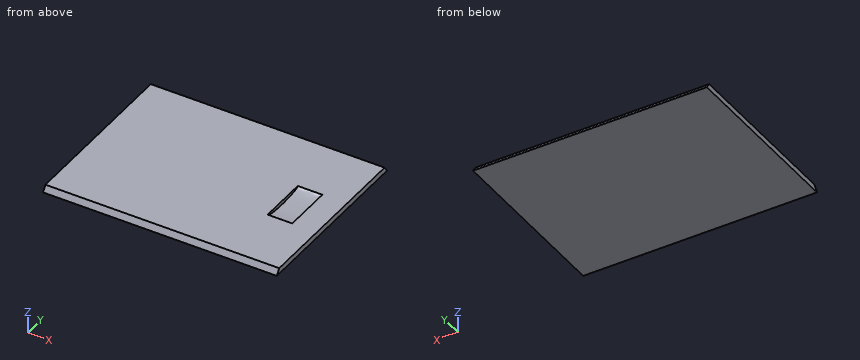
from build123d import *

# Parameters (mm, degrees)
ESBO_O1_W                = 4.6
ESBO_O1_H                = 140
RESSALTO_EXTRUS_O1_DEPTH = 190
CORTE_EXTRUS_O1_START    = -20
ESBO_O2_RX               = 20.00007904
ESBO_O2_RY               = 3.000011856
CORTE_EXTRUS_O1_DEPTH    = 20


with BuildPart() as part:
    # Esboço1 → Ressalto-extrusão1 (new body)
    with BuildSketch(Plane(origin=(0, 0, 0), x_dir=(0, 0, -1), z_dir=(1, 0, 0))):
        Rectangle(ESBO_O1_W, ESBO_O1_H)
        Polygon((2.3, 70), (-2.3, 70), (2.3, 73.220954676), align=None)
        Polygon((2.3, -70), (-2.3, -70), (2.3, -73.220954676), align=None)
    extrude(amount=RESSALTO_EXTRUS_O1_DEPTH)

    # Esboço2 → Corte-extrusão1 (cut)
    with BuildSketch(Plane(origin=(190, 0, 0), x_dir=(0, 0, -1), z_dir=(1, 0, 0)).offset(CORTE_EXTRUS_O1_START)):
        with Locations(Location((-2.3, 0), (0, 0, -89.838918547))):
            Ellipse(ESBO_O2_RX, ESBO_O2_RY)
    extrude(amount=-CORTE_EXTRUS_O1_DEPTH, mode=Mode.SUBTRACT)


solid = part.part
CAD build for the part. Positions are in the model's coordinates, mm. Round coordinates to 2 decimals unless told otherwise and drop trailing zeros. Write each loop counter-clockwise with the first axis right and the second up, starting at its lowest first coordinate (ties: lowest second). Pieces come first, ordered by that corner, then holes. Notation, with made-up numbers: M 74,28.25 L 108,28.25 A14 cw 108,48.25 Z; hole C 40.25,24 d10. An arc over 180 degrees is marked long. Use a Markdown table: item, result. Add a question column.
1. Drill centre lines: probe 1 along Y at (x, z) = (26, 1.55); probe 2 along Y at (x, z) = (123.5, 1.05); probe 3 along Z at (x, y) = (164.5, 10.5). Where is each one in solid material? Low to high.
2. Flat gauge pin, fed straight in: P1, Ø2, axis at x = 67.5, z = 0, coming from the +Y side. Where does the tip first touch, or does it go through?
3. Slice it at A-A on x = 127. Give the cut face in (y, z), then the cut area to 3 significant figures.
Reply:
| question | item | result |
|---|---|---|
| 1 | probe 1 | y = -70.53 to 70.53 |
| 1 | probe 2 | y = -70.88 to 70.88 |
| 1 | probe 3 | z = -2.3 to -0.22 |
| 2 | P1 | stops at y = 72.31 |
| 3 | outline | M -73.22,-2.3 L 73.22,-2.3 L 70,2.3 L -70,2.3 Z |
| 3 | area | 659 mm^2 |
